from build123d import *

# Parameters (mm, degrees)
SKETCH2_R                                           = 60.625
SKETCH2_R_2                                         = 45
BOSS_EXTRUDE1_DEPTH                                 = 4.5
SKETCH3_R                                           = 49
SKETCH3_R_2                                         = 45
BOSS_EXTRUDE2_DEPTH                                 = 52
SKETCH4_W                                           = 13.25
SKETCH4_H                                           = 8
SKETCH4_W_2                                         = 8
SKETCH4_H_2                                         = 38.5
BOSS_EXTRUDE3_DEPTH                                 = 13
SKETCH5_W                                           = 10
SKETCH5_H                                           = 20
CUT_EXTRUDE1_DEPTH                                  = 26
SKETCH6_R                                           = 5
CUT_EXTRUDE2_DEPTH                                  = 110.698023
SKETCH7_R                                           = 1.3
CUT_EXTRUDE3_DEPTH                                  = 7.2
BOSS_EXTRUDE4_DEPTH                                 = 4
CSK_FOR_M3_COUNTERSUNK_FLAT_HEAD_SCREW1_D           = 3.4
CSK_FOR_M3_COUNTERSUNK_FLAT_HEAD_SCREW1_DEPTH       = 44.45
CSK_FOR_M3_COUNTERSUNK_FLAT_HEAD_SCREW1_CSINK_D     = 6.3
CSK_FOR_M3_COUNTERSUNK_FLAT_HEAD_SCREW1_CSINK_ANGLE = 90
CSK_FOR_M3_COUNTERSUNK_FLAT_HEAD_SCREW1_TIP         = 1.021463052
FILLET1_R                                           = 1


with BuildPart() as part:
    # Sketch2 → Boss-Extrude1 (new body)
    with BuildSketch(Plane(origin=(0, 0, 0), x_dir=(1, 0, 0), z_dir=(0, 1, 0))):
        with Locations(Location((0, 0, 0), (0, 0, 270))):
            Circle(SKETCH2_R)
        with Locations(Location((0, 0, 0), (0, 0, 270))):
            Circle(SKETCH2_R_2, mode=Mode.SUBTRACT)
    extrude(amount=BOSS_EXTRUDE1_DEPTH)

    # Sketch3 → Boss-Extrude2 (add)
    with BuildSketch(Plane(origin=(0, 4.5, 0), x_dir=(1, 0, 0), z_dir=(0, 1, 0))):
        with Locations(Location((0, 0, 0), (0, 0, 90))):
            Circle(SKETCH3_R)
        with Locations(Location((0, 0, 0), (0, 0, 270))):
            Circle(SKETCH3_R_2, mode=Mode.SUBTRACT)
    extrude(amount=BOSS_EXTRUDE2_DEPTH)

    # Sketch4 → Boss-Extrude3 (add, symmetric)
    with BuildSketch(Plane(origin=(0, 0, 0), x_dir=(0, 0, -1), z_dir=(1, 0, 0))):
        Polygon((-31.75, 30.5), (-45, 30.5), (-45, 17.25), align=None)
        with Locations((-38.375, 34.5)):
            Rectangle(SKETCH4_W, SKETCH4_H)
        with Locations((15.25, 19.25)):
            Rectangle(SKETCH4_W_2, SKETCH4_H_2)
    extrude(amount=BOSS_EXTRUDE3_DEPTH, both=True)


with BuildPart() as boss_extrude3_piece_1:
    # of the separate pieces the step leaves, piece 1, a body of its own (boss_extrude3_pieces)
    add(part.part.solids().sort_by_distance((0, 0, 60.625))[0])


with BuildPart() as boss_extrude3_piece_2:
    # of the separate pieces the step leaves, piece 2, a body of its own (boss_extrude3_pieces)
    add(part.part.solids().sort_by_distance((-13, 38.5, -19.25))[0])

    # Sketch5 → Cut-Extrude1 (cut)
    with BuildSketch(Plane.XY):
        with Locations((0, 19.5)):
            Rectangle(SKETCH5_W, SKETCH5_H)
    extrude(amount=-CUT_EXTRUDE1_DEPTH, mode=Mode.SUBTRACT)


with BuildPart() as cut_extrude2_tool:
    # Sketch6 → Cut-Extrude2 (new, through all)
    with BuildSketch(Plane.XY.offset(-11.25)):
        with Locations(Location((0, 14, 0), (0, 0, 90))):
            Circle(SKETCH6_R)
    extrude(amount=-CUT_EXTRUDE2_DEPTH)


with BuildPart() as boss_extrude3_piece_1_1:
    add(boss_extrude3_piece_1.part)

    # Cut-Extrude2: cut by cut_extrude2_tool
    add(cut_extrude2_tool.part, mode=Mode.SUBTRACT)


with BuildPart() as boss_extrude3_piece_2_1:
    add(boss_extrude3_piece_2.part)

    # Cut-Extrude2: cut by cut_extrude2_tool
    add(cut_extrude2_tool.part, mode=Mode.SUBTRACT)


with BuildPart() as cut_extrude3_tool:
    # Sketch7 → Cut-Extrude3 (new body)
    with BuildSketch(Plane(origin=(0, 38.5, 0), x_dir=(1, 0, 0), z_dir=(0, 1, 0))):
        with Locations(Location((-5, 13.75, 0), (0, 0, 270))):
            Circle(SKETCH7_R)
        with Locations(Location((5, 13.75, 0), (0, 0, 270))):
            Circle(SKETCH7_R)
        with Locations(Location((-5, -34.25, 0), (0, 0, 270))):
            Circle(SKETCH7_R)
        with Locations(Location((5, -34.25, 0), (0, 0, 270))):
            Circle(SKETCH7_R)
    extrude(amount=-CUT_EXTRUDE3_DEPTH)


with BuildPart() as boss_extrude3_piece_1_2:
    add(boss_extrude3_piece_1_1.part)

    # Cut-Extrude3: cut by cut_extrude3_tool
    add(cut_extrude3_tool.part, mode=Mode.SUBTRACT)



with BuildPart() as boss_extrude3_piece_2_2:
    add(boss_extrude3_piece_2_1.part)

    # Cut-Extrude3: cut by cut_extrude3_tool
    add(cut_extrude3_tool.part, mode=Mode.SUBTRACT)


with BuildPart() as boss_extrude3_piece_1_3:
    add(boss_extrude3_piece_1_2.part)

    add(boss_extrude3_piece_2_2.part)  # Boss-Extrude4 merges Boss-Extrude3 piece 2
    # Sketch8 → Boss-Extrude4 (add)
    with BuildSketch(Plane.XZ):
        with BuildLine():
            Line((13, -11.25), (-13, -11.25))
            Line((-13, -11.25), (-37.248431585, -25.249838503))
            ThreePointArc((-37.248431585, -25.249838503), (0, -45), (37.248431585, -25.249838503))
            Line((37.248431585, -25.249838503), (13, -11.25))
        make_face()
        with BuildLine():
            Line((-19.516660498, -24.25), (-24.906460381, -27.361802413))
            ThreePointArc((-24.906460381, -27.361802413), (0, -37), (24.906460381, -27.361802413))
            Line((24.906460381, -27.361802413), (19.516660498, -24.25))
            Line((19.516660498, -24.25), (-19.516660498, -24.25))
        make_face(mode=Mode.SUBTRACT)
    extrude(amount=-BOSS_EXTRUDE4_DEPTH)

    # CSK for M3 Countersunk Flat Head Screw1
    with Locations(Plane(origin=(-35, 4.5, -42), x_dir=(0, 0, 1), z_dir=(0, 1, 0))):
        with Locations((0, 0), (0, 70), (84, 70), (84, 0)):
            CounterSinkHole(CSK_FOR_M3_COUNTERSUNK_FLAT_HEAD_SCREW1_D / 2, CSK_FOR_M3_COUNTERSUNK_FLAT_HEAD_SCREW1_CSINK_D / 2, depth=CSK_FOR_M3_COUNTERSUNK_FLAT_HEAD_SCREW1_DEPTH, counter_sink_angle=CSK_FOR_M3_COUNTERSUNK_FLAT_HEAD_SCREW1_CSINK_ANGLE)
            with Locations((0, 0, -(CSK_FOR_M3_COUNTERSUNK_FLAT_HEAD_SCREW1_DEPTH + CSK_FOR_M3_COUNTERSUNK_FLAT_HEAD_SCREW1_TIP / 2))):  # 118° drill point
                Cone(0, CSK_FOR_M3_COUNTERSUNK_FLAT_HEAD_SCREW1_D / 2, CSK_FOR_M3_COUNTERSUNK_FLAT_HEAD_SCREW1_TIP, mode=Mode.SUBTRACT)

    # Fillet1
    fillet1_edges = [boss_extrude3_piece_1_3.edges().sort_by_distance(p)[0] for p in [
        (0, 4.5, 49),
    ]]
    fillet(fillet1_edges, radius=FILLET1_R)


solid = boss_extrude3_piece_1_3.part
Check sheet for the modelled part. Datum: model origin and axes. Units: mm. A direction names the side the tool comes from. Give positions to 0.01 mm unless a question says otherwise; leave off trailing zeros. Write each loop counter-clockwise with the first axis right and the second up, starting at its lowest first coordinate (ties: lowest second). Pieces come first, ordered by that corner, then holes. Notation, with made-up numbers: (12.25, 61) -> (24.25, 61) arc R14 ccw to (24.25, 77) -> close; hole circle Ø8 at (38, -9.75). An arc over 180 degrees is marked (long way). One line per item, written item: value. Start each with the question number.
Item 1: Section check B-B on x = 0. State how many separate pieces and enclosed holes the cut face has, then the cut area to 3 significant figures.
Item 2: Gauge pin test, flat ends, axial feed: pin 1 (9 mm diameter, centred on x = 5.5, z = -15, fed in from +Y); pin 2 (3 mm diameter, centred on y = 38, z = -6.5, fed in from -X); pin 3 (1.5 mm diameter, centred on y = 46, z = -15.5, fed in from -X); pin 4 (5 mm diameter, centred on x = 24, z = -14.5, fed in from -Y). Record the tip position at first contact, or that the pin passes through.
Item 3: Draft check along Y on faces 1 (the flat face through (-0.18, 23.78, 38.47)), 2 (the cylindrical face through (33.97, 1.5, -40.65)), 3 (the flat face through (-1, 4, -24)), 4 (the flat face through (-4, 9.5, -15)). Enter one of: +Y half, -Y half, draft (parallel to the pull), parting line (faces both ways), or undercut.
Item 4: Section check A-A on y = 21.5. Record the cut outline in (x, z), then the cut area to 3 significant figures.
Item 5: Tool access check on faces 5 (the flat face through (4, 9.5, -15)), 6 (the cylindrical face through (0, 9, -15)), 7 (the flat face through (-24.95, 1.97, -18.15)), 8 (the flat face through (13, 21, -15)). Record the directions out of +Z, -Z, +X, -X, +Y, -Y that give a thin tool (end or side, any length) a straight path to the whole face; none if there is none.
Item 6: Material ranges on probe 1 along X at (y, z) = (1.25, -42); probe 2 along Z at (x, y) = (12.5, 25); probe 3 along Z at (x, y) = (35, 1.8), recorded low to high. Write a range as from..to.
Item 7: Section check C-C on z = 0. Record the cut outline in (x, y) (3 decimals).
Item 8: Section check D-D on y = 11.5. Record the cut outline in (x, z).
Results list:
1. separate pieces: 5
1. enclosed holes: 0
1. area: 907 mm²
2. pin 1: y = 38.5
2. pin 2: x = -48.74
2. pin 3: x = -46.73
2. pin 4: through
3. face 1: -Y half
3. face 2: draft
3. face 3: +Y half
3. face 4: undercut
4. outline: circle Ø98 at (0, 0); (-13, -19.25) -> (-5, -19.25) -> (-5, -11.25) -> (-13, -11.25) -> close; (5, -19.25) -> (13, -19.25) -> (13, -11.25) -> (5, -11.25) -> close; hole (-13, 40.75) -> (-13, 43.08) arc R45 ccw (long way) to (13, 43.08) -> (13, 40.75) -> close
4. area: 1,400 mm²
5. face 5: none
5. face 6: -Z
5. face 7: +Y, -Y
5. face 8: +Y
6. probe 1: -43.72..-36.7, -33.3..33.3, 36.7..43.72
6. probe 2: -47.38..-43.23, -19.25..-11.25, 37.25..47.38
6. probe 3: -49.5..-43.7, -40.3..-23.95, 28.28..40.3, 43.7..49.5
7. outline: (-60.625, 0) -> (-45, 0) -> (-45, 56.5) -> (-49, 56.5) -> (-49, 5.5) arc R1 cw to (-50, 4.5) -> (-60.625, 4.5) -> close; (45, 0) -> (60.625, 0) -> (60.625, 4.5) -> (50, 4.5) arc R1 cw to (49, 5.5) -> (49, 56.5) -> (45, 56.5) -> close
8. outline: (-13, -19.25) -> (-5, -19.25) -> (-5, -11.25) -> (-13, -11.25) -> close; (-4.33, -48.81) -> (-4.33, -44.79) arc R45 cw (long way) to (4.33, -44.79) -> (4.33, -48.81) arc R49 ccw (long way) to start; (5, -19.25) -> (13, -19.25) -> (13, -11.25) -> (5, -11.25) -> close
